from build123d import *

# Parameters (mm, degrees)
SKETCH1_W           = 28
SKETCH1_H           = 27
BOSS_EXTRUDE1_DEPTH = 8
SKETCH2_R           = 1.48371595
CUT_EXTRUDE1_DEPTH  = 22.029740845
SKETCH3_R           = 3
CUT_EXTRUDE2_DEPTH  = 3
FILLET1_R           = 2.5
SKETCH4_R           = 2.5
CUT_EXTRUDE3_DEPTH  = 11.5
SKETCH5_R           = 4
CUT_EXTRUDE4_DEPTH  = 14


with BuildPart() as part:
    # Sketch1 → Boss-Extrude1 (new body)
    with BuildSketch(Plane.XY):
        Rectangle(SKETCH1_W, SKETCH1_H)
    extrude(amount=BOSS_EXTRUDE1_DEPTH)

    # Sketch2 → Cut-Extrude1 (cut, through all)
    with BuildSketch(Plane.XY.offset(8)):
        with Locations((-6.5, 8.5)):
            Circle(SKETCH2_R)
        with Locations((-6.5, -8.5)):
            Circle(SKETCH2_R)
        with Locations((8, -7)):
            Circle(SKETCH2_R)
        with Locations((8, 7)):
            Circle(SKETCH2_R)
    extrude(amount=-CUT_EXTRUDE1_DEPTH, mode=Mode.SUBTRACT)

    # Sketch3 → Cut-Extrude2 (cut)
    with BuildSketch(Plane.XY.offset(8)):
        with Locations((-6.5, 8.5)):
            Circle(SKETCH3_R)
        with Locations((8, -7)):
            Circle(SKETCH3_R)
        Polygon((-8.112712507, -11.2933), (-4.887287493, -11.2933), (-3.274574986, -8.5), (-4.887287493, -5.7067), (-8.112712507, -5.7067), (-9.725425014, -8.5), align=None)
        Polygon((6.387287493, 4.2067), (9.612712507, 4.2067), (11.225425014, 7), (9.612712507, 9.7933), (6.387287493, 9.7933), (4.774574986, 7), align=None)
    extrude(amount=-CUT_EXTRUDE2_DEPTH, mode=Mode.SUBTRACT)

    # Fillet1
    fillet1_edges = [part.edges().sort_by_distance(p)[0] for p in [
        (-14, 13.5, 4),
        (14, 13.5, 4),
        (14, -13.5, 4),
        (-14, -13.5, 4),
    ]]
    fillet(fillet1_edges, radius=FILLET1_R)

    # Sketch4 → Cut-Extrude3 (cut)
    with BuildSketch(Plane(origin=(14, 0, 0), x_dir=(0, 0, -1), z_dir=(1, 0, 0))):
        with Locations((0.5, 0)):
            Circle(SKETCH4_R)
    extrude(amount=-CUT_EXTRUDE3_DEPTH, mode=Mode.SUBTRACT)

    # Sketch5 → Cut-Extrude4 (cut)
    with BuildSketch(Plane.ZY.offset(14)):
        with Locations((-0.5, 0)):
            Circle(SKETCH5_R)
    extrude(amount=-CUT_EXTRUDE4_DEPTH, mode=Mode.SUBTRACT)


solid = part.part
Check sheet for the modelled part. Datum: model origin and axes. Units: mm. A direction names the side the tool comes from. Round coordinates to 2 decimals unless told otherwise and drop trailing zeros. Loops run counter-clockwise (first coordinate to the right, second up) from the corner with the lowest first, then second, coordinate; pieces in that order, holes last.
1. Sectioned sample at A-A on x = 8. Record the boundary of the cut face in (y, z), and give its area (3 significant figures).
2. Scan lines: probe 1 along Y at (x, z) = (8, 6.8); probe 2 along X at (y, z) = (-7.75, 4.5); probe 3 along Y at (x, z) = (8, 1.7). Record each from-to range of solid material in increasing order.
3. Gauge pin test, flat ends, axial feed: pin 1 Ø1.6 at (y, z) = (0, 0.5) entering from +X; pin 2 Ø1.8 at (y, z) = (0.5, 1) entering from -X; pin 3 Ø3.5 at (x, y) = (-6.5, -8.5) entering from +Z. Record the tip position at first contact, or that the pin passes through.
4. Set-up check for faces 1 (the cylindrical face through (8, 0, 2)), 2 (the cylindrical face through (-7.1, -0.1, 3.5)), 3 (the flat face through (-5, -7, 5)): record each of +Z, -Z, +X, -X, +Y, -Y from which the full face is reachable in a straight line by a thin tool's end or side.
5. Sectioned sample at C-C on y = 6.5. Record the boundary of the cut face in (x, z), and give its area (3 significant figures).
6. Sectioned sample at D-D on y = 2. Record the boundary of the cut face in (x, z), and give its area (3 significant figures).
7. Mould release check, pull along Y, two halves, no side actions. Record for faces 4 (the flat face through (0, 13.5, 4)), 5 (the flat face through (14, 0, 4)), 6 (the flat face through (-8.908, -7.084, 6.521)), 7 (the flat face through (-8.93, -9.88, 6.52)): released by +Y, released by -Y, zero draft, split by the parting line, or undercut.
8. Sectioned sample at B-B on z = 4.25. Record the boundary of the cut face in (x, y).
Recorded:
1. outline: (-13.5, 0) - (-8.48, 0) - (-8.48, 5) - (-10, 5) - (-10, 8) - (-13.5, 8) - close; (-5.52, 0) - (-2.45, 0) arc R2.5 cw to (2.45, 0) - (5.52, 0) - (5.52, 5) - (4.21, 5) - (4.21, 8) - (-4, 8) - (-4, 5) - (-5.52, 5) - close; (8.48, 0) - (13.5, 0) - (13.5, 8) - (9.79, 8) - (9.79, 5) - (8.48, 5) - close
1. area: 144 mm2
2. probe 1: y = -13.5 to -10, -4 to 4.21, 9.79 to 13.5
2. probe 2: x = -14 to -7.78, -5.22 to 6.72, 9.28 to 14
2. probe 3: y = -13.5 to -8.48, -5.52 to -1.19, 1.19 to 5.52, 8.48 to 13.5
3. pin 1: stops at x = 2.5
3. pin 2: stops at x = 0
3. pin 3: stops at z = 5
4. face 1: -Z, +X
4. face 2: -Z, -X
4. face 3: +Z
5. outline: (-14, 0) - (6.6, 0) - (6.6, 5) - (5.06, 5) - (5.06, 8) - (-4.26, 8) - (-4.26, 5) - (-8.74, 5) - (-8.74, 8) - (-14, 8) - close; (9.4, 0) - (14, 0) - (14, 8) - (10.94, 8) - (10.94, 5) - (9.4, 5) - close
5. area: 179 mm2
6. outline: (-14, 2.96) - (0, 2.96) - (0, 0) - (2.5, 0) - (2.5, 1) - (14, 1) - (14, 8) - (-14, 8) - close
6. area: 171 mm2
7. face 4: released by +Y
7. face 5: zero draft
7. face 6: undercut
7. face 7: undercut
8. outline: (-14, -11) arc R2.5 ccw to (-11.5, -13.5) - (11.5, -13.5) arc R2.5 ccw to (14, -11) - (14, 11) arc R2.5 ccw to (11.5, 13.5) - (-11.5, 13.5) arc R2.5 ccw to (-14, 11) - close; hole circle Ø2.97 at (-6.5, -8.5); hole circle Ø2.97 at (-6.5, 8.5); hole circle Ø2.97 at (8, -7); hole circle Ø2.97 at (8, 7)
